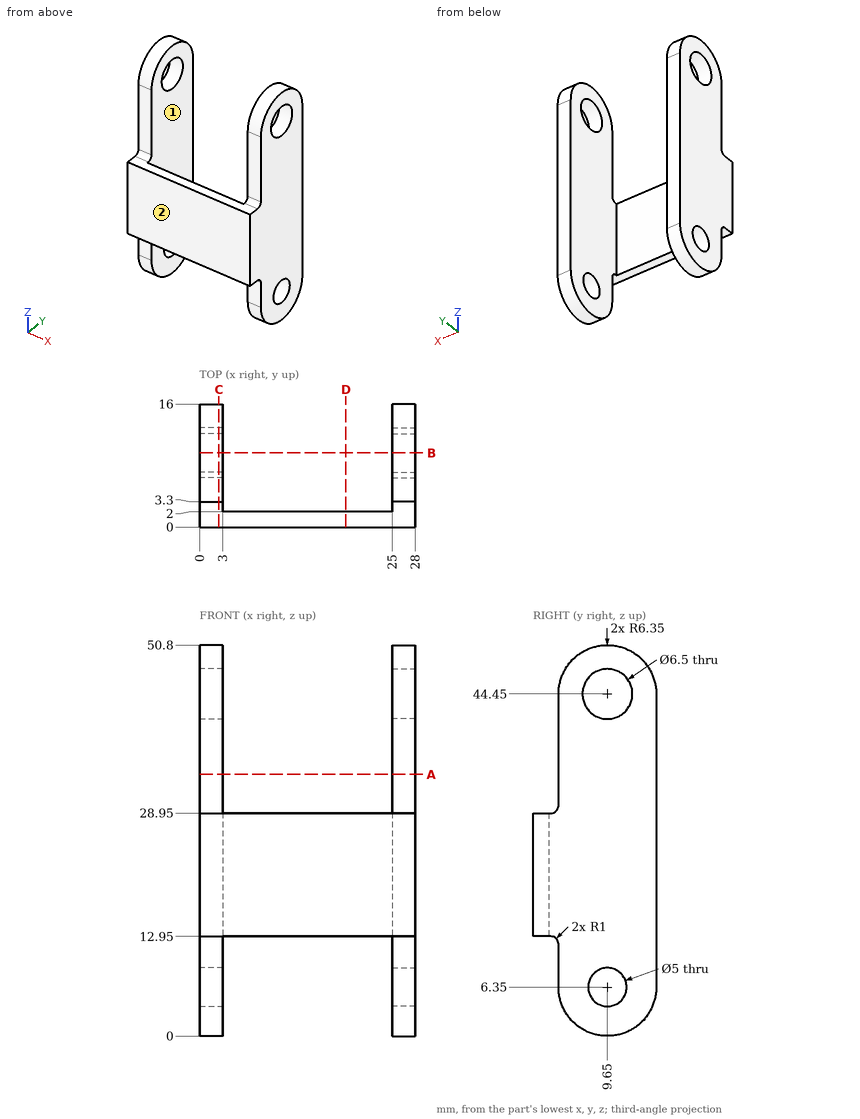
Geometry check sheet. Reference: drawing and pictorial views, mm from the part's lowest x, y, z. A direction names the side the tool comes from. Give positions to 0.01 mm unless a question says otherwise; leave off trailing zeros. Loops run counter-clockwise (first coordinate to the right, second up) from the corner with the lowest first, then second, coordinate; pieces in that order, holes last. Notation, with made-up numbers: (63.25, 80) - (104.25, 80) arc R12 ccw to (104.25, 98) - close; hole circle Ø4 at (51.25, -15). An arc over 180 degrees is marked (long way). One line per question, with ' | ' between items. Start each with the question number.
1. Material ranges on line 1 along X through (y, z) = (5.5, 20); line 2 along Y through (x, z) = (26.25, 44.45); line 3 along Z through (x, y) = (9.5, 1.5), recorded low to high. Write a range as [from, to].
2. Gauge pin test, flat ends, axial feed: pin 1 Ø1.2 at (x, y) = (8, 0.5) entering from -Z; pin 2 Ø8 at (x, y) = (20.5, 7) entering from +Z; pin 3 Ø3.5 at (x, z) = (2, 34) entering from -Y; pin 4 Ø1.8 at (x, y) = (17.5, 0.5) entering from +Z. Record the tip position at first contact, or that the pin passes through.
3. Cross-section at C-C, the plane x = 2.5. Enter the section's corners in (y, z).
4. Set-up check for the marked faces 1 and 2: record each of +Z, -Z, +X, -X, +Y, -Y from which the full face is reachable in a straight line by a thin tool's end or side.
5. Cross-section at D-D, the plane x = 19. Enter the section's corners in (y, z).
6. Cross-section at A-A, the plane z = 34. Enter the section's corners in (x, y), plus the area to 3 significant figures.
7. Cross-section at B-B, the plane y = 9.65. Enter the section's corners in (x, z).
Check result:
1) line 1: x = [0, 3], [25, 28] | line 2: y = [3.3, 6.4], [12.9, 16] | line 3: z = [12.95, 28.95]
2) pin 1: stops at z = 12.95 | pin 2: passes through | pin 3: stops at y = 3.3 | pin 4: stops at z = 28.95
3) outline: (0, 12.95) - (2.3, 12.95) arc R1 cw to (3.3, 11.95) - (3.3, 6.35) arc R6.35 ccw to (16, 6.35) - (16, 44.45) arc R6.35 ccw to (3.3, 44.45) - (3.3, 29.95) arc R1 cw to (2.3, 28.95) - (0, 28.95) - close; hole circle Ø6.5 at (9.65, 44.45); hole circle Ø5 at (9.65, 6.35)
4) face 1: +Z, -Z, +Y | face 2: +Z, -Z, +X, -X, -Y
5) outline: (0, 12.95) - (2, 12.95) - (2, 28.95) - (0, 28.95) - close
6) outline: (0, 3.3) - (3, 3.3) - (3, 16) - (0, 16) - close; (25, 3.3) - (28, 3.3) - (28, 16) - (25, 16) - close | area: 76.2 mm2
7) outline: (0, 0) - (3, 0) - (3, 3.85) - (0, 3.85) - close; (0, 8.85) - (3, 8.85) - (3, 41.2) - (0, 41.2) - close; (0, 47.7) - (3, 47.7) - (3, 50.8) - (0, 50.8) - close; (25, 0) - (28, 0) - (28, 3.85) - (25, 3.85) - close; (25, 8.85) - (28, 8.85) - (28, 41.2) - (25, 41.2) - close; (25, 47.7) - (28, 47.7) - (28, 50.8) - (25, 50.8) - close
